from build123d import *

# Parameters (mm, degrees)
CROQUIS1_R              = 2.5
SALIENTE_EXTRUIR1_DEPTH = 44.1
REDONDEO1_SIZE          = 0.5
SKETCH_1_W              = 5.27274558
SKETCH_1_H              = 1.959781543
CUT_EXTRUDE_1_DEPTH     = 17.5


with BuildPart() as part:
    # Croquis1 → Saliente-Extruir1 (new body)
    with BuildSketch(Plane.XY):
        Circle(CROQUIS1_R)
    extrude(amount=SALIENTE_EXTRUIR1_DEPTH)

    # Redondeo1
    redondeo1_edges = [part.edges().sort_by_distance(p)[0] for p in [
        (-2.5, 0, 44.1),
    ]]
    chamfer(redondeo1_edges, length=REDONDEO1_SIZE)

    # Эскиз1 → Вырез-Вытянуть1 (cut)
    with BuildSketch(Plane.XY.offset(44.1)):
        with Locations((0.092224381, 2.979890772)):
            Rectangle(SKETCH_1_W, SKETCH_1_H)
    extrude(amount=-CUT_EXTRUDE_1_DEPTH, mode=Mode.SUBTRACT)


solid = part.part
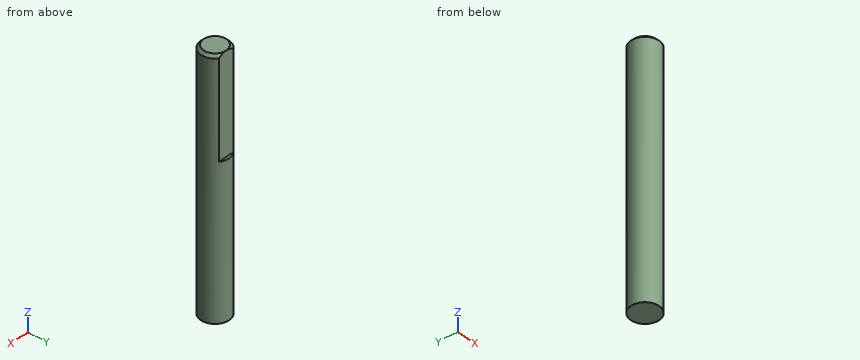
The listing builds one solid part. Answer for the finished solid, in the listing's coordinates (mm). Give positions to 0.01 mm unless a question says otherwise; leave off trailing zeros. Write each loop counter-clockwise with the first axis right and the second up, starting at its lowest first coordinate (ties: lowest second). Pieces come first, ordered by that corner, then holes. Notation, with made-up numbers: (9.25, 8.25) - (17.25, 8.25) arc R18 cw to (17.25, 35.25) - close; hole circle Ø5 at (18.25, -14). An arc over 180 degrees is marked (long way). Use a Markdown table: item, result.
1. Section B-B on z = 18 is taken. Write down the section's boundary in (x, y).
Values follow:
| item | result |
|---|---|
| outline | circle Ø5 at (0, 0) |
2. Find the intervals of material crossed by probe 1 along X at (y, z) = (1.25, 13); probe 2 along X at (y, z) = (-0.8, 24); probe 3 along Y at (x, z) = (1, 42.5), in increasing order. Write a range as from..to.
Values follow:
| item | result |
|---|---|
| probe 1 | x = -2.17..2.17 |
| probe 2 | x = -2.37..2.37 |
| probe 3 | y = -2.29..2 |
3. Section A-A on z = 36.5 is taken. Write down the section's boundary in (x, y).
Values follow:
| item | result |
|---|---|
| outline | (-1.5, 2) arc R2.5 ccw (long way) to (1.5, 2) - close |
4. Each of these flat-tipped pins is pushed along its axis until it touches: P1, Ø1.5, axis at x = -1.5, z = 4.5, coming from the -Y side; P2, Ø3, axis at x = -0.5, z = 33, coming from the +Y side. Where does it stop, or does it pass through?
Values follow:
| item | result |
|---|---|
| P1 | stops at y = -2.38 |
| P2 | stops at y = 2 |
